Source: CAD feature listing. Evaluate the final solid. Frame: model axes, mm. Round coordinates to 2 decimals unless told otherwise and drop trailing zeros. Order: outer loops, then holes, each group sorted by start corner. A loop starts at its lowest first (then second) coordinate and runs counter-clockwise, first axis right, second up. Notation, with made-up numbers: (12, 6) -> (42, 6) arc R26 ccw to (42, 21) -> close; hole circle Ø9 at (29.25, 12). An arc over 180 degrees is marked (long way). One line per item, written item: value. Start each with the question number.
1) Section B-B (z = 134.5). Return the cut outline in (x, y).
2) Ray query, L1, parallel to Z at x = 172.5, y = 1.1; L2, parallel to X at y = 2.85, z = 139.5; L3, parallel to X at y = 1.1, z = -90. Return the intervals inside material, ascending.
3) Pin query (flat end, axial travel): P1, Ø4, axis at x = 172.5, z = -172.5, coming from the -Y side. Return the tip coordinate at first contact, or that it passes through.
4) Section A-A (x = 267.5). Return the cut outline in (y, z).
```python
from build123d import *

# Parameters (mm, degrees)
SKETCH1_W               = 595
SKETCH1_H               = 395
BOSS_EXTRUDE1_DEPTH     = 3
CUT_EXTRUDE1_DEPTH      = 10
CUT_EXTRUDE2_DEPTH      = 358.10152618
CUT_EXTRUDE2_DEPTH_BACK = 358.10152618
SKETCH5_W               = 3.3
SKETCH5_H               = 389
CUT_EXTRUDE3_DEPTH      = 358.10152618
CUT_EXTRUDE3_DEPTH_BACK = 358.10152618
SKETCH6_R               = 2.6


with BuildPart() as part:
    # Sketch1 → Boss-Extrude1 (new body)
    with BuildSketch(Plane(origin=(0, 0, 0), x_dir=(1, 0, 0), z_dir=(0, 1, 0))):
        Rectangle(SKETCH1_W, SKETCH1_H)
    extrude(amount=BOSS_EXTRUDE1_DEPTH)

    # Sketch2 → Cut-Extrude1 (cut)
    with BuildSketch(Plane(origin=(0, 3, 0), x_dir=(1, 0, 0), z_dir=(0, 1, 0))):
        with BuildLine():
            Line((275, -112.5), (275, -142.5))
            ThreePointArc((275, -142.5), (267.5, -150), (260, -142.5))
            Line((260, -142.5), (260, -112.5))
            ThreePointArc((260, -112.5), (267.5, -105), (275, -112.5))
        make_face()
    extrude(amount=-CUT_EXTRUDE1_DEPTH, mode=Mode.SUBTRACT)

    # Sketch5 → Cut-Extrude2 (cut, two sides: drawn at the far end of the back side and taken through both)
    with BuildSketch(Plane(origin=(0, 3, 0), x_dir=(1, 0, 0), z_dir=(0, 1, 0)).offset(-CUT_EXTRUDE2_DEPTH_BACK)):
        with Locations((-291, 0)):
            Rectangle(SKETCH5_W, SKETCH5_H)
        with Locations((291, 0)):
            Rectangle(SKETCH5_W, SKETCH5_H)
    extrude(amount=CUT_EXTRUDE2_DEPTH + CUT_EXTRUDE2_DEPTH_BACK, mode=Mode.SUBTRACT)

    # Sketch6 → Cut-Extrude3 (cut, two sides: drawn at the far end of the back side and taken through both)
    with BuildSketch(Plane(origin=(0, 3, 0), x_dir=(1, 0, 0), z_dir=(0, 1, 0)).offset(-CUT_EXTRUDE3_DEPTH_BACK)):
        with Locations(Location((172.5, 172.5, 0), (0, 0, 270))):
            Circle(SKETCH6_R)
        with Locations(Location((-172.5, -172.5, 0), (0, 0, 270))):
            Circle(SKETCH6_R)
        with Locations(Location((172.5, -172.5, 0), (0, 0, 270))):
            Circle(SKETCH6_R)
        with Locations(Location((-172.5, 172.5, 0), (0, 0, 270))):
            Circle(SKETCH6_R)
    extrude(amount=CUT_EXTRUDE3_DEPTH + CUT_EXTRUDE3_DEPTH_BACK, mode=Mode.SUBTRACT)


solid = part.part
```
Findings:
1. outline: (-297.5, 0) -> (-292.65, 0) -> (-292.65, 3) -> (-297.5, 3) -> close; (-289.35, 0) -> (260, 0) -> (260, 3) -> (-289.35, 3) -> close; (275, 0) -> (289.35, 0) -> (289.35, 3) -> (275, 3) -> close; (292.65, 0) -> (297.5, 0) -> (297.5, 3) -> (292.65, 3) -> close
2. L1: -197.5 to -175.1, -169.9 to 169.9, 175.1 to 197.5
2. L2: -297.5 to -292.65, -289.35 to 260, 275 to 289.35, 292.65 to 297.5
2. L3: -297.5 to -292.65, -289.35 to 289.35, 292.65 to 297.5
3. P1: through
4. outline: (0, -197.5) -> (3, -197.5) -> (3, 105) -> (0, 105) -> close; (0, 150) -> (3, 150) -> (3, 197.5) -> (0, 197.5) -> close
